Autodesk Inventor part; units mm, degrees
ref_plane "YZ Plane" through (0, 0, 0) normal (1, 0, 0) x (0, 1, 0)
ref_plane "XZ Plane" through (0, 0, 0) normal (0, 1, 0) x (-1, 0, 0)
ref_plane "XY Plane" through (0, 0, 0) normal (0, 0, 1) x (1, 0, 0)
sketch "Sketch1" plane through (0, 0, 0) normal (0, 1, 0) x (-1, 0, 0)
  line L0 (-3.1474, 0) -> (12.0926, 0)
  line L1 (12.0926, 0) -> (12.0926, -23.222)
  line L2 (12.0926, -23.222) -> (34.9526, -23.222)
  line L3 (34.9526, -25) -> (9.5526, -25)
  line L4 (9.5526, -25) -> (9.5526, -1.778)
  line L5 (9.5526, -1.778) -> (-3.1474, -1.778)
  line L6 (-3.1474, -1.778) -> (-3.1474, 0)
  line L7 (34.9526, -25) -> (34.9526, -23.222)
  dimension "d1" = 1.778
  dimension "d2" = 25
  dimension "d3" = 1.778
  dimension "d5" = 25.4
  dimension "d6" = 2.54
  dimension "d26" = 15.24
extrude "Extrusion1" add sketch "Sketch1" along normal mid plane 25.4
sketch "Sketch2" plane through (-34.9526, 12.7, -23.222) normal (0, 0, 1) x (1, 0, 0)
  arc A0 (12.0273, -25.4) -> (12.0273, 0) centre (-9.5066, -12.7) ccw
  line L0 (0, 0) -> (12.0273, 0)
  line L1 (12.1267, -25.23) -> (0, -25.23)
  line L2 (0, -25.23) -> (0, 0)
  line L3 (11.8723, 0) -> (11.8723, -12.7) construction
  line L4 (11.8723, -12.7) -> (11.8723, -25.4) construction
  line L5 (22.86, -25.4) -> (0, -25.4) construction
  line L6 (11.8723, -12.7) -> (-9.5066, -12.7) construction
  line L7 (0, 0) -> (0, -25.4) construction
  point P0 (34.9526, -12.7)
  dimension "d9" = 50
extrude "Extrusion2" add sketch "Sketch2" along normal blind 3.7
sketch "Sketch3" plane through (3.1474, 12.7, -1.778) normal (0, 0, -1) x (-1, 0, 0)
  line L0 (0, -25.4) -> (0, 0)
  line L1 (0, -15.8818) -> (33.02, -25.4)
  line L2 (38.1, -25.4) -> (12.7, -25.4)
  line L3 (0, -25.4) -> (0, -15.8818)
  line L4 (0, -25.4) -> (33.02, -25.4)
  point P0 (3.1474, -12.7)
  point P1 (0, 0)
  dimension "d12" = 73.92
  dimension "d13" = 33.02
extrude "Extrusion3" cut sketch "Sketch3" along normal mid plane 76.2
sketch "Sketch4" plane through (3.1474, 12.7, -1.778) normal (0, 0, -1) x (-1, 0, 0)
  line L0 (0, -15.8818) -> (0, -8.9488) construction
  line L1 (0, 0) -> (0, -15.8818) construction
  line L2 (2.54, -8.9488) -> (2.54, -2.4488) construction
  line L3 (0, -8.9488) -> (2.54, -8.9488) construction
  point P0 (3.1474, -12.7)
  dimension "d16" = 6.933
  dimension "d17" = 2.54
  dimension "d18" = 6.5
hole "Hole1" at (0.6074, 3.7512, -1.778) at (0.6074, 10.2512, -1.778) direction (0, 0, 1) diameter 3 end through all
sketch "Sketch5" plane through (-34.9526, 12.7, -19.522) normal (0, 0, 1) x (1, 0, 0)
  circle A0 centre (6.8106, -12.7) radius 3.175
  point P0 (34.9526, -12.7)
  dimension "d28" = 6.35
extrude "Extrusion4" cut sketch "Sketch5" against normal blind 3.81
sketch "Sketch6" plane through (-28.1421, 0, -23.332) normal (0, 0, 1) x (1, 0, 0)
  line L0 (-0.0036, 0) -> (1.7744, 0)
  line L1 (-0.0036, 0) -> (-1.7816, 0)
  point P0 (28.1421, 0)
  dimension "d31" = 1.778
hole "Hole2" at (-29.9236, 0, -23.332) at (-26.3676, 0, -23.332) direction (0, 0, -1) diameter 1.5 end through all
sketch "Sketch7" plane through (-12.0926, 12.7, -23.222) normal (-1, 0, 0) x (0, 0, 1)
  line L0 (23.222, -20.2748) -> (21.444, -20.2748)
  line L1 (21.444, -20.2748) -> (21.444, 0)
  line L2 (21.444, 0) -> (23.222, 0)
  line L3 (23.222, 0) -> (23.222, -20.2748)
  point P0 (23.222, -12.7)
extrude "Extrusion5" add sketch "Sketch7" along normal blind 10.16
sketch "Sketch8" plane through (-12.0926, -7.5748, -1.778) normal (0, 0, -1) x (-1, 0, 0)
  line L0 (0, 20.2748) -> (10.16, 20.2748)
  line L1 (10.16, 0) -> (7.62, 0)
  line L2 (7.62, 0) -> (7.62, 20.2748)
  line L3 (7.62, 20.2748) -> (10.16, 20.2748)
  line L4 (10.16, 20.2748) -> (10.16, 0)
  point P0 (-12.0926, 7.5748)
  dimension "d43" = 2.54
extrude "Extrusion6" add sketch "Sketch8" along normal blind 5.08
sketch "Sketch9" plane through (-22.2526, 12.7, -23.222) normal (-1, 0, 0) x (0, 0, 1)
  line L0 (0, -20.2748) -> (21.444, -20.2748)
  line L1 (16.364, 0) -> (18.904, 0)
  line L2 (18.904, 0) -> (18.904, -20.2748)
  line L3 (18.904, -20.2748) -> (16.364, -20.2748)
  line L4 (16.364, -20.2748) -> (16.364, 0)
  point P0 (23.222, -12.7)
  dimension "d44" = 2.54
extrude "Extrusion7" add sketch "Sketch9" along normal blind 10.16
sketch "Sketch10" plane through (-12.0926, -7.5748, -6.858) normal (0, 0, -1) x (-1, 0, 0)
  line L0 (16.002, 20.2748) -> (16.002, 7.5748)
  line L1 (16.002, 7.5748) -> (14.224, 7.5748)
  line L2 (7.62, 20.2748) -> (16.002, 20.2748) construction
  line L3 (7.62, 20.2748) -> (7.62, 0) construction
  line L4 (16.002, 7.5748) -> (17.78, 7.5748)
  point P0 (-12.0926, 7.5748)
  point P1 (20.32, 20.2748)
  dimension "d47" = 1.778
  dimension "d48" = 8.382
  dimension "d49" = 12.7
hole "Hole3" at (-26.3166, 0, -6.858) at (-29.8726, 0, -6.858) direction (0, 0, 1) diameter 1.5 end through all
properties part number "Encoder Mount v2"
CAD build for the part. Positions are in the model's coordinates, mm. A direction names the side the tool comes from. Coordinates: 2 decimals unless noted, no trailing zeros. Write each loop counter-clockwise with the first axis right and the second up, starting at its lowest first coordinate (ties: lowest second). Pieces come first, ordered by that corner, then holes. Notation, with made-up numbers: (-3.75, 26.5) -> (33.25, 26.5) arc R15 ccw to (33.25, 37.5) -> close; hole circle Ø5 at (-17, 79). An arc over 180 degrees is marked (long way). Use CSV: the item, a comma, the result in double quotes. Start each with the question number.
Item 1: Tool access for faces 1 (the flat face through (-32.413, 3, -6)), 2 (the cylindrical face through (-25.635, 0.163, -24.178)), 3 (the flat face through (-26, 2, -6.858)), 4 (the flat face through (-19.713, 2, -4)): list every direction of +Z, -Z, +X, -X, +Y, -Y with a clear straight run to the whole face (end or side of a thin tool).
Item 2: Band-saw the part on C-C, the plane z = -21.5. Write the cut outline in (x, y) (3 decimals).
Item 3: Band-saw the part on D-D, the plane y = 4. Write the cut outline in (x, z).
Item 4: Two-plate mould, pull along Y, no slides. Class faces 5 (the cylindrical face through (0.157, 5.182, -0.877)), 6 (the cylindrical face through (-29.2, 0.2, -24.2)), 7 (the flat face through (-32, -12.53, -21)), 8 (the flat face through (-9.553, 3, -14)): +Y half, -Y half, draft (parallel to the pull), parting line (faces both ways), or undercut.
Item 5: Band-saw the part on B-B, the plane x = -24.5. Write the cut outline in (y, z), plus the area to 3 significant figures.
Item 6: Drop flat-ended pins along their axis: P1, Ø5, axis at x = -25.5, y = 4.5, coming from the +Z side; P2, Ø1, axis at x = -26.5, z = -21.5, coming from the -Y side; P3, Ø2, axis at y = -4, z = -6.5, coming from the -X side; P4, Ø2.5, axis at x = 0.61, y = 3.75, coming from the +Z side. Give the stop position or say it passes through.
Item 7: Band-saw the part on A-A, the plane z = -2.25. Write the cut outline in (x, y), plus the area to 3 significant figures.
Item 8: Wall check: probe 1 along X at (y, z) = (0, -5); probe 2 along Z at (x, y) = (-15, 0); probe 3 along Z at (x, y) = (-29, 5.75). Give the ranges that are in metal, low to high.
Response values:
1,face 1,"+Z, -X, +Y, -Y"
1,face 2,"-Z"
1,face 3,"-X, +Y, -Y"
1,face 4,"+Y, -Y"
2,outline,"(-34.953, -12.53) -> (-29.283, -12.53) -> (-21.7, -10.344) arc R25 ccw to (-22.925, 12.7) -> (-34.953, 12.7) -> close; (-12.093, -7.575) -> (-9.553, -6.843) -> (-9.553, 12.7) -> (-12.093, 12.7) -> close; hole circle Ø6.35 at (-28.142, 0)"
3,outline,"(-34.95, -25) -> (-9.55, -25) -> (-9.55, -1.78) -> (-0.87, -1.78) -> (-0.87, 0) -> (-22.25, 0) -> (-22.25, -4.32) -> (-32.41, -4.32) -> (-32.41, -6.86) -> (-19.71, -6.86) -> (-19.71, -1.78) -> (-12.09, -1.78) -> (-12.09, -23.22) -> (-19.78, -23.22) -> (-19.78, -19.52) -> (-34.95, -19.52) -> close; (2.09, -1.78) -> (3.15, -1.78) -> (3.15, 0) -> (2.09, 0) -> close"
4,face 5,"undercut"
4,face 6,"undercut"
4,face 7,"-Y half"
4,face 8,"draft"
5,outline,"(-11.15, -25) -> (12.7, -25) -> (12.7, -19.52) -> (-11.15, -19.52) -> close; (-7.57, -6.86) -> (12.7, -6.86) -> (12.7, -4.32) -> (-7.57, -4.32) -> close"
5,area,"182 mm2"
6,P1,"stops at z = -4.32"
6,P2,"stops at y = -11.87"
6,P3,"stops at x = -32.41"
6,P4,"passes through"
7,outline,"(-22.25, -7.57) -> (-19.71, -7.57) -> (-19.71, 12.7) -> (-22.25, 12.7) -> close; (-12.09, -7.57) -> (-9.55, -6.84) -> (-9.55, 12.7) -> (-12.09, 12.7) -> close"
7,area,"102 mm2"
8,probe 1,"x = -32.41 to -30.62, -29.12 to -27.07, -25.57 to -19.71, -12.09 to -9.55"
8,probe 2,"z = -25 to -23.22, -1.78 to 0"
8,probe 3,"z = -25 to -19.52, -6.86 to -4.32"
